from build123d import *

# Parameters (mm, degrees)
SZKIC1_W                    = 60
SZKIC1_H                    = 120
SZKIC1_R                    = 2.75
SZKIC1_R_2                  = 3.6
SZKIC1_R_3                  = 10.25
SZKIC1_R_4                  = 1.75
DODANIE_WYCI_GNI_CIE1_DEPTH = 4
ZAOKR_GLENIE1_R             = 4
SZKIC2_W                    = 1.4
SZKIC2_H                    = 6
WYTNIJ_WYCI_GNI_CIE1_DEPTH  = 10
ZAOKR_GLENIE2_R             = 1
ZAOKR_GLENIE3_R             = 1


with BuildPart() as part:
    # Szkic1 → Dodanie-wyciągnięcie1 (new body)
    with BuildSketch(Plane.XY):
        with Locations((19.115931961, 35.506335127)):
            Rectangle(SZKIC1_W, SZKIC1_H)
        with Locations((-0.884068039, 45.706335127)):
            Circle(SZKIC1_R, mode=Mode.SUBTRACT)
        with Locations((-0.884068039, -14.493664873)):
            Circle(SZKIC1_R_2, mode=Mode.SUBTRACT)
        with Locations((39.115931961, -14.493664873)):
            Circle(SZKIC1_R_2, mode=Mode.SUBTRACT)
        with Locations((39.115931961, 45.706335127)):
            Circle(SZKIC1_R, mode=Mode.SUBTRACT)
        with Locations((19.115931961, 80.506335127)):
            Circle(SZKIC1_R_3, mode=Mode.SUBTRACT)
        with Locations((6.298755985, 87.906335127)):
            Circle(SZKIC1_R_4, mode=Mode.SUBTRACT)
        with Locations((31.933107937, 87.906335127)):
            Circle(SZKIC1_R_4, mode=Mode.SUBTRACT)
        with Locations((19.115931961, 65.706335127)):
            Circle(SZKIC1_R_4, mode=Mode.SUBTRACT)
    extrude(amount=DODANIE_WYCI_GNI_CIE1_DEPTH)

    # Zaokrąglenie1
    zaokr_glenie1_edges = [part.edges().sort_by_distance(p)[0] for p in [
        (-10.884068039, 95.506335127, 2),
        (49.115931961, 95.506335127, 2),
        (49.115931961, -24.493664873, 2),
        (-10.884068039, -24.493664873, 2),
    ]]
    fillet(zaokr_glenie1_edges, radius=ZAOKR_GLENIE1_R)

    # Szkic2 → Wytnij-wyciągnięcie1 (cut)
    with BuildSketch(Plane.XY.offset(4)):
        with Locations((-7.184068039, 15.606335127)):
            Rectangle(SZKIC2_W, SZKIC2_H)
        Polygon((-10.884068039, 21.606335127), (-7.884068039, 18.606335127), (-6.484068039, 18.606335127), (-10.884068039, 23.006335127), align=None)
        Polygon((49.115931961, 23.006335127), (44.715931961, 18.606335127), (46.115931961, 18.606335127), (49.115931961, 21.606335127), align=None)
        with Locations((45.415931961, 15.606335127)):
            Rectangle(SZKIC2_W, SZKIC2_H)
    extrude(amount=-WYTNIJ_WYCI_GNI_CIE1_DEPTH, mode=Mode.SUBTRACT)

    # Zaokrąglenie2
    zaokr_glenie2_edges = [part.edges().sort_by_distance(p)[0] for p in [
        (49.115931961, 21.606335127, 2),
        (49.115931961, 23.006335127, 2),
    ]]
    fillet(zaokr_glenie2_edges, radius=ZAOKR_GLENIE2_R)

    # Zaokrąglenie3
    zaokr_glenie3_edges = [part.edges().sort_by_distance(p)[0] for p in [
        (-10.884068039, 23.006335127, 2),
        (-10.884068039, 21.606335127, 2),
    ]]
    fillet(zaokr_glenie3_edges, radius=ZAOKR_GLENIE3_R)


solid = part.part
The model under review builds one solid part; all positions refer to its coordinate system, in mm. A direction names the side the tool comes from. Round coordinates to 2 decimals unless told otherwise and drop trailing zeros. Write each loop counter-clockwise with the first axis right and the second up, starting at its lowest first coordinate (ties: lowest second). Pieces come first, ordered by that corner, then holes. Notation, with made-up numbers: (37, 56.25) - (51, 56.25) arc R27 cw to (51, 78.25) - close; hole circle Ø1 at (-5.5, -8.75). An arc over 180 degrees is marked (long way). One line per item, written item: value. Start each with the question number.
1. Consider section A-A on y = 72. Write out the cut boundary in (x, z).
2. Consider section C-C on z = 1.55. State how many separate pieces and enclosed holes the cut face has, and give its area (3 significant figures).
3. To check wall thickness, follow L1, parallel to Y at x = -1, z = 0.55; L2, parallel to Y at x = 39.5, z = 3.35; L3, parallel to X at y = 87, z = 0.6. State the ranges of each line that lie inside material, in increasing order. Write a range as from..to.
4. The part is to be moulded in two halves that separate along Y. For faces 1 (the face through (49.116, 57, 2)), 2 (the face through (-9.743, 94.303, 2.028)), 3 (the face through (-7.884, 16, 2)), say which applies: released by +Y, released by -Y, zero draft, split by the parting line, or undercut.
5. Machinability: for faces 4 (the face through (46.116, 16, 2)), 5 (the face through (19, 36, 0)), which of the approach directions +Z, -Z, +X, -X, +Y, -Y give a long, thin tool a straight path to every point of the face, cutting with its end or side? Answer none if there is none.
6. Consider section B-B on x = 15. Write out the cut boundary in (y, z), and give its area (3 significant figures).
Checks:
1. outline: (-10.88, 0) - (13.4, 0) - (13.4, 4) - (-10.88, 4) - close; (24.83, 0) - (49.12, 0) - (49.12, 4) - (24.83, 4) - close
2. separate pieces: 1
2. enclosed holes: 8
2. area: 6,670 mm^2
3. L1: y = -24.49..-18.09, -10.9..42.96, 48.45..95.51
3. L2: y = -24.49..-18.07, -10.91..42.98, 48.43..95.51
3. L3: x = -10.88..4.8, 7.8..11.19, 27.05..30.44, 33.43..49.12
4. face 1: zero draft
4. face 2: released by +Y
4. face 3: undercut
5. face 4: +Z, -Z
5. face 5: -Z, +X, -X, +Y, -Y
6. outline: (-24.49, 0) - (71.12, 0) - (71.12, 4) - (-24.49, 4) - close; (89.89, 0) - (95.51, 0) - (95.51, 4) - (89.89, 4) - close
6. area: 405 mm^2
